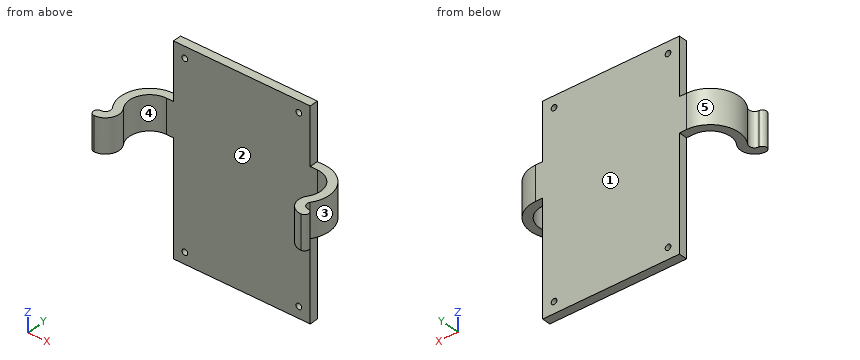
```python
from build123d import *

# Parameters (mm, degrees)
F1_DEPTH = 19.05
F2_W     = 76.2
F2_H     = 31.75
F2_H_2   = 63.5
F3_DEPTH = 4.7625
F4_R     = 1.5875
F5_DEPTH = 4.7625


with BuildPart() as f1:
    # F0 (on Top) → F1 (new body)
    with BuildSketch(Plane.XY):
        with BuildLine():
            ThreePointArc((42.037, 11.303), (52.118297, 5.111287), (51.154651, -6.680288))
            ThreePointArc((51.154651, -6.680288), (50.904065, -14.490744), (57.600453, -18.518697))
            ThreePointArc((57.600453, -18.518697), (60.007424, -16.163448), (57.652175, -13.756478))
            ThreePointArc((57.652175, -13.756478), (55.11432, -12.262843), (55.124148, -9.318092))
            ThreePointArc((55.124148, -9.318092), (56.316357, 7.362081), (42.037, 16.0655))
            Line((42.037, 16.0655), (0, 16.0655))
            Line((0, 16.0655), (-42.037, 16.0655))
            ThreePointArc((-42.037, 16.0655), (-56.316357, 7.362081), (-55.124148, -9.318092))
            ThreePointArc((-55.124148, -9.318092), (-55.11432, -12.262843), (-57.652175, -13.756478))
            ThreePointArc((-57.652175, -13.756478), (-60.007424, -16.163448), (-57.600453, -18.518697))
            ThreePointArc((-57.600453, -18.518697), (-50.904065, -14.490744), (-51.154651, -6.680288))
            ThreePointArc((-51.154651, -6.680288), (-52.118297, 5.111287), (-42.037, 11.303))
            Line((-42.037, 11.303), (0, 11.303))
            Line((0, 11.303), (42.037, 11.303))
        make_face()
    extrude(amount=F1_DEPTH)

    # F2 (on face) → F3 (join)
    with BuildSketch(Plane(origin=(0, 16.0655, 0), x_dir=(-1, 0, 0), z_dir=(0, 1, 0))):
        with Locations((0, 34.925)):
            Rectangle(F2_W, F2_H)
        with Locations((0, -31.75)):
            Rectangle(F2_W, F2_H_2)
    extrude(amount=-F3_DEPTH)

    # F4 (on face) → F5 (cut)
    with BuildSketch(Plane(origin=(0, 16.0655, 0), x_dir=(-1, 0, 0), z_dir=(0, 1, 0))):
        with Locations((-31.75, 44.45)):
            Circle(F4_R)
        with Locations((31.75, 44.45)):
            Circle(F4_R)
        with Locations((31.75, -57.15)):
            Circle(F4_R)
        with Locations((-31.75, -57.15)):
            Circle(F4_R)
    extrude(amount=-F5_DEPTH, mode=Mode.SUBTRACT)


solid = f1.part
```
Source: CAD feature listing. Evaluate the final solid. Frame: model axes, mm. Face numbers are marked on the shaded views. A direction names the side the tool comes from. Coordinates: 2 decimals unless noted, no trailing zeros. Order: outer loops, then holes, each group sorted by start corner. A loop starts at its lowest first (then second) coordinate and runs counter-clockwise, first axis right, second up. Notation, with made-up numbers: M 71,81 L 87,81 A22 ccw 87,97 Z; hole C 68,42.25 d2. An arc over 180 degrees is marked long. Write each question's results on one line, items separated by ' | '. Start each with the question number.
1) Section query B-B (y = 0.5). Return the cut outline in (x, z).
2) Line query: line 1 (Z direction, x = 31.75, y = 14.6); line 2 (X direction, y = 14, z = -57); line 3 (Y direction, x = 10, z = 23). Output: solid intervals per line, ascending. Write a range as from..to.
3) Access query for the marked faces 4 and 5. Directions: +Z, -Z, +X, -X, +Y, -Y. A direction counts if a zero-diameter tool reaches every point of the face in a straight line with its end or side. Return the directions, or none.
4) Contact query for flat-ended pins moving along their axis: pin 1 Ø4 at (x, z) = (-31.75, -57.15) entering from -Y; pin 2 Ø1 at (y, z) = (12, -12) entering from +X; pin 3 Ø17.5 at (x, y) = (-46, 4) entering from +Z. Output: stop coordinate, or through.
5) Section query D-D (x = 3). Return the cut outline in (y, z).
6) Draft query along X for the marked faces 1, 2 and 3. Return one class per face: released by +X, released by -X, zero draft, split by the parting line, or undercut.
7) Section query A-A (z = -57.15). Return the cut outline in (x, y).
8) Section query C-C (x = 31.75). Return the cut outline in (y, z), plus the area to 3 significant figures.
Answers:
1) outline: M -58.09,0 L -53.33,0 L -53.33,19.05 L -58.09,19.05 Z; M 53.33,0 L 58.09,0 L 58.09,19.05 L 53.33,19.05 Z
2) line 1: z = -63.5..-58.74, -55.56..42.86, 46.04..50.8 | line 2: x = -38.1..-33.33, -30.17..30.17, 33.33..38.1 | line 3: y = 11.3..16.07
3) face 4: +Z, -Z | face 5: +Z, -Z, -X
4) pin 1: stops at y = 11.3 | pin 2: stops at x = 38.1 | pin 3: stops at z = 19.05
5) outline: M 11.3,-63.5 L 16.07,-63.5 L 16.07,50.8 L 11.3,50.8 Z
6) face 1: zero draft | face 2: undercut | face 3: released by +X
7) outline: M -38.1,11.3 L -33.34,11.3 L -33.34,16.07 L -38.1,16.07 Z; M -30.16,11.3 L 30.16,11.3 L 30.16,16.07 L -30.16,16.07 Z; M 33.34,11.3 L 38.1,11.3 L 38.1,16.07 L 33.34,16.07 Z
8) outline: M 11.3,-63.5 L 16.07,-63.5 L 16.07,-58.74 L 11.3,-58.74 Z; M 11.3,-55.56 L 16.07,-55.56 L 16.07,42.86 L 11.3,42.86 Z; M 11.3,46.04 L 16.07,46.04 L 16.07,50.8 L 11.3,50.8 Z | area: 514 mm^2
